Part model, mm, in its own coordinate system. A direction names the side the tool comes from. Coordinates: 2 decimals unless noted, no trailing zeros. Loops run counter-clockwise (first coordinate to the right, second up) from the corner with the lowest first, then second, coordinate; pieces in that order, holes last. Notation, with made-up numbers: (88, 21) - (102, 21) arc R18 cw to (102, 27) - close; hole circle Ø6 at (58.25, 9.25). An arc over 180 degrees is marked (long way). Use a Markdown table: item, result. Add a question column.
1. Pull direction X, two halves, no side cores. Call faces 1 (the flat face through (10, 20, 5)), 2 (the cylindrical face through (18.699, 1.285, 5.437)), 3 (the flat face through (20, 10, 5)): pulls with the +X half, pulls with the -X half, needs draft (parallel to the pull), parting line crosses it, or undercut.
2. Wall check: probe 1 along Y at (x, z) = (14, 5); probe 2 along Z at (x, y) = (1.5, 3.25). Give the ranges that are in metal, low to high. Write a range as [from, to].
3. Drop a flat-ended pin along its axis: pin 1 (2 mm diameter, centred on x = 15.5, y = 5, fed in from +Z). Give the stop position or say it passes through.
4. Band-saw the part on A-A, the plane z = 5. Give the cut face in (x, y), plus the area to 3 significant figures.
5. 3-axis set-ups, long thin cutter, end or side, ignore diameter. For faces 4 (the flat face through (10, 10, 0)), 5 (the flat face through (9, 1, 6)): which of +Z, -Z, +X, -X, +Y, -Y reach the whole face in a straight line?
6. Band-saw the part on B-B, the plane x = 10. Give the cut face in (y, z).
from build123d import *

# Parameters (mm, degrees)
SKETCH_W     = 20
SKETCH_H     = 20
PAD_DEPTH    = 10
SKETCH001_W  = 18
SKETCH001_H  = 18
POCKET_DEPTH = 9
FILLET_R     = 1
FILLET001_R  = 1


with BuildPart() as part:
    # Sketch → Pad (new body)
    with BuildSketch(Plane.XY):
        with Locations((10, 10)):
            Rectangle(SKETCH_W, SKETCH_H)
    extrude(amount=PAD_DEPTH)

    # Sketch001 → Pocket (cut)
    with BuildSketch(Plane.XY.offset(10)):
        with Locations((10, 10)):
            Rectangle(SKETCH001_W, SKETCH001_H)
    extrude(amount=-POCKET_DEPTH, mode=Mode.SUBTRACT)

    # Fillet
    fillet_edges = [part.edges().sort_by_distance(p)[0] for p in [
        (20, 0, 5),
    ]]
    fillet(fillet_edges, radius=FILLET_R)

    # Fillet001
    fillet001_edges = [part.edges().sort_by_distance(p)[0] for p in [
        (19, 1, 5.5),
    ]]
    fillet(fillet001_edges, radius=FILLET001_R)


solid = part.part
Geometry check:
| question | item | result |
|---|---|---|
| 1 | face 1 | needs draft |
| 1 | face 2 | undercut |
| 1 | face 3 | pulls with the +X half |
| 2 | probe 1 | y = [0, 1], [19, 20] |
| 2 | probe 2 | z = [0, 1] |
| 3 | pin 1 | stops at z = 1 |
| 4 | outline | (0, 0) - (19, 0) arc R1 ccw to (20, 1) - (20, 20) - (0, 20) - close; hole (1, 1) - (18, 1) arc R1 ccw to (19, 2) - (19, 19) - (1, 19) - close |
| 4 | area | 76.0 mm^2 |
| 5 | face 4 | -Z, +X, -X, +Y, -Y |
| 5 | face 5 | +Z |
| 6 | outline | (0, 0) - (20, 0) - (20, 10) - (19, 10) - (19, 1) - (1, 1) - (1, 10) - (0, 10) - close |
